The listing builds one solid part. Answer for the finished solid, in the listing's coordinates (mm). Round coordinates to 2 decimals unless told otherwise and drop trailing zeros. Loops run counter-clockwise (first coordinate to the right, second up) from the corner with the lowest first, then second, coordinate; pieces in that order, holes last. Notation, with made-up numbers: (28.25, -22.75) -> (64.25, -22.75) arc R34 cw to (64.25, 14.25) -> close; hole circle Ø1 at (78, 28). An arc over 180 degrees is marked (long way). Write each question's results on one line, items separated by ' | '. Start each with the question number.
(1) The part is cut by section B-B (z = 3.5). Determine the outline of the cut face in (x, y).
(2) Straight lines are drawn through the part: probe 1 along Y at (x, z) = (0, 10); probe 2 along X at (y, z) = (0, 16.25); probe 3 along Y at (x, z) = (-50, 13). For each, find the intervals that lie inside material, in ascending order.
(3) Determine the mould class of faces 1 (the face through (76.2, -1, 18)), 2 (the face through (16, 1, 25.4)), 3 (the face through (-76.2, 1, 18)), 4 (the face through (12.114, 3.815, 12.878)) for opening direction X: released by +X, released by -X, zero draft, split by the parting line, or undercut.
(4) The part is cut by section A-A (x = 0). Determine the outline of the cut face in (y, z).
(5) A flat-ended cylindrical pin translates along its axis: pin 1 (3 mm diameter, centred on x = 56, y = -16.5, fed in from -Z). Find the tip coordinate at first contact, or state that the pin passes through.
```python
from build123d import *

# Parameters (mm, degrees)
F1_DEPTH = 25.4
F2_R     = 12.7
F3_DEPTH = 25.401
F5_DEPTH = 152.401


with BuildPart() as f1:
    # F0 (on Top) → F1 (new body)
    with BuildSketch(Plane.XY):
        with BuildLine():
            Line((69.85, 50.8), (-69.85, 50.8))
            ThreePointArc((-69.85, 50.8), (-74.340128, 48.940128), (-76.2, 44.45))
            Line((-76.2, 44.45), (-76.2, -44.45))
            ThreePointArc((-76.2, -44.45), (-74.340128, -48.940128), (-69.85, -50.8))
            Line((-69.85, -50.8), (69.85, -50.8))
            ThreePointArc((69.85, -50.8), (74.340128, -48.940128), (76.2, -44.45))
            Line((76.2, -44.45), (76.2, 44.45))
            ThreePointArc((76.2, 44.45), (74.340128, 48.940128), (69.85, 50.8))
        make_face()
    extrude(amount=F1_DEPTH)

    # F2 (on face) → F3 (cut, through all)
    with BuildSketch(Plane.XY.offset(25.4)):
        Circle(F2_R)
    extrude(amount=-F3_DEPTH, mode=Mode.SUBTRACT)

    # F4 (on face) → F5 (cut, through all)
    with BuildSketch(Plane(origin=(-76.2, 0, 0), x_dir=(0, -1, 0), z_dir=(-1, 0, 0))):
        with BuildLine():
            ThreePointArc((-3.175, 12.7), (-2.245064, 10.454936), (0, 9.525))
            Line((0, 9.525), (0, 12.7))
            Line((0, 12.7), (-3.175, 12.7))
        make_face()
        with BuildLine():
            Line((0, 12.7), (0, 9.525))
            ThreePointArc((0, 9.525), (2.245064, 10.454936), (3.175, 12.7))
            ThreePointArc((3.175, 12.7), (2.245064, 14.945064), (0, 15.875))
            Line((0, 15.875), (0, 12.7))
        make_face()
        with BuildLine():
            Line((-3.175, 12.7), (0, 12.7))
            Line((0, 12.7), (0, 15.875))
            ThreePointArc((0, 15.875), (-2.245064, 14.945064), (-3.175, 12.7))
        make_face()
    extrude(amount=-F5_DEPTH, mode=Mode.SUBTRACT)


solid = f1.part
```
Checked values:
1) outline: (-76.2, -44.45) arc R6.35 ccw to (-69.85, -50.8) -> (69.85, -50.8) arc R6.35 ccw to (76.2, -44.45) -> (76.2, 44.45) arc R6.35 ccw to (69.85, 50.8) -> (-69.85, 50.8) arc R6.35 ccw to (-76.2, 44.45) -> close; hole circle Ø25.4 at (0, 0)
2) probe 1: y = -50.8 to -12.7, 12.7 to 50.8 | probe 2: x = -76.2 to -12.7, 12.7 to 76.2 | probe 3: y = -50.8 to -3.16, 3.16 to 50.8
3) face 1: released by +X | face 2: zero draft | face 3: released by -X | face 4: undercut
4) outline: (-50.8, 0) -> (-12.7, 0) -> (-12.7, 25.4) -> (-50.8, 25.4) -> close; (12.7, 0) -> (50.8, 0) -> (50.8, 25.4) -> (12.7, 25.4) -> close
5) pin 1: stops at z = 0
